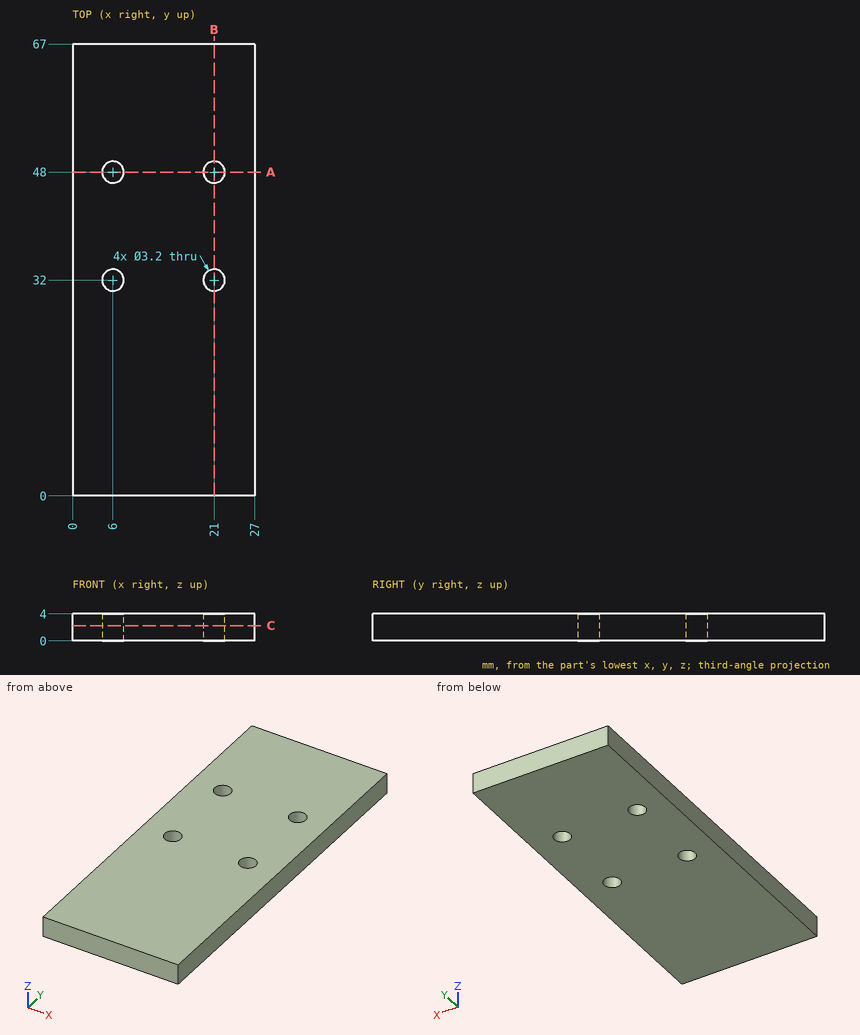
Can you work these out from the drawing? Everything is in mm from the part's minimum corner. Coordinates: 2 decimals unless noted, no trailing zeros. Loops run counter-clockwise (first coordinate to the right, second up) from the corner with the lowest first, then second, coordinate; pieces in that order, holes last.
1. Imagine slicing it at A-A, the plane y = 48. Please give me the cut outline in (x, z).
2. For P1, Ø6, axis at x = 10.5, y = 9.5, coming from the -Z side, with a flat end and sliding along its axis, tell me the tip position at first contact or that it passes through.
3. Imagine slicing it at B-B, the plane x = 21. Please give me the cut outline in (y, z), and give its area (3 significant figures).
4. Imagine slicing it at C-C, the plane z = 2.25. Please give me the cut outline in (x, y).
5. I need wall thicknesses on L1, parallel to Y at x = 21, z = 2.1; L2, parallel to X at y = 31.5, z = 1.9. Which ranges of each line are inside material? Lowest first, please.
Taken from the geometry:
1. outline: (0, 0) - (4.4, 0) - (4.4, 4) - (0, 4) - close; (7.6, 0) - (19.4, 0) - (19.4, 4) - (7.6, 4) - close; (22.6, 0) - (27, 0) - (27, 4) - (22.6, 4) - close
2. P1: stops at z = 0
3. outline: (0, 0) - (30.4, 0) - (30.4, 4) - (0, 4) - close; (33.6, 0) - (46.4, 0) - (46.4, 4) - (33.6, 4) - close; (49.6, 0) - (67, 0) - (67, 4) - (49.6, 4) - close
3. area: 242 mm2
4. outline: (0, 0) - (27, 0) - (27, 67) - (0, 67) - close; hole circle Ø3.2 at (6, 32); hole circle Ø3.2 at (6, 48); hole circle Ø3.2 at (21, 32); hole circle Ø3.2 at (21, 48)
5. L1: y = 0 to 30.4, 33.6 to 46.4, 49.6 to 67
5. L2: x = 0 to 4.48, 7.52 to 19.48, 22.52 to 27
